```python
from build123d import *

# Parameters (mm, degrees)
F3_D           = 6.2
F3_CSINK_D     = 11
F3_CSINK_ANGLE = 90


with BuildPart() as f1:
    # F0 (on Top) → F1 (revolve)
    with BuildSketch(Plane.XY):
        Polygon((0, 11), (0, 0), (12, 0), (12, 6), (10.5, 6), (9, 4.5), (7.5, 6), (4, 6), (4, 11), align=None)
    revolve(axis=Axis((6, 0, 0), (1, 0, 0)))

    # F3 (through all)
    with Locations(Plane.YZ.offset(12)):
        with Locations((0, 0)):
            CounterSinkHole(F3_D / 2, F3_CSINK_D / 2, counter_sink_angle=F3_CSINK_ANGLE)


solid = f1.part
```
For this review, take the finished solid that the model builds, in its own axes (mm). A direction names the side the tool comes from. Coordinates: 2 decimals unless noted, no trailing zeros. Write each loop counter-clockwise with the first axis right and the second up, starting at its lowest first coordinate (ties: lowest second). Pieces come first, ordered by that corner, then holes. Notation, with made-up numbers: (-27, -30.75) - (-21, -30.75) arc R4 ccw to (-21, -26.75) - close; hole circle Ø5 at (48, 75.25). An arc over 180 degrees is marked (long way). Answer in a Markdown table with one row per item. Add a question column.
Q1. For P1, Ø1.5, axis at y = -4, z = 6.5, coming from the +X side; P2, Ø5.5, axis at y = 0, z = 0, coming from the -X side; P3, Ø1, axis at x = 3, y = 2.5, coming from the -Z side, all flat-tipped, find the tip position at first contact; note any pin that passes through.
Q2. Tool access review of faces 1 (the cylindrical face through (1.97, -2.38, -10.74)), 2 (the cylindrical face through (11, -6, 0)): name each direction out of +Z, -Z, +X, -X, +Y, -Y from which nothing blocks a thin tool from reaching the whole face with its end or side.
Q3. We need section D-D, the plane x = 8. State the section outline as (y, z) points.
Q4. We need section A-A, the plane y = 0. State the section outline as (x, z) points, and give its area (3 significant figures).
Q5. Draft analysis for pull direction Y (two halves, no side actions). For faces 3 (the cylindrical face through (6, -6, 0)), 4 (the conical face through (9.717, 0.697, -3.14)), 5 (the flat face through (12, -3, -5)), state which applies: +Y half, -Y half, draft (parallel to the pull), parting line (faces both ways), or undercut.
Q6. We need section C-C, the plane x = 3.25. State the section outline as (y, z) points, and give its area (3 significant figures).
Q7. For probe 1 along Z at (x, y) = (3, 0); probe 2 along Z at (x, y) = (5.25, 0); probe 3 along X at (y, z) = (-5.75, -6.5), list the stretches that pass through material, from the lowest coordinate up.
Answer list:
| question | item | result |
|---|---|---|
| 1 | P1 | stops at x = 4 |
| 1 | P2 | passes through |
| 1 | P3 | stops at z = -10.82 |
| 2 | face 1 | +X, -X |
| 2 | face 2 | +X |
| 3 | outline | circle Ø11 at (0, 0); hole circle Ø6.2 at (0, 0) |
| 4 | outline | (0, -11) - (4, -11) - (4, -6) - (7.5, -6) - (9, -4.5) - (10.5, -6) - (12, -6) - (12, -5.5) - (9.6, -3.1) - (0, -3.1) - close; (0, 3.1) - (9.6, 3.1) - (12, 5.5) - (12, 6) - (10.5, 6) - (9, 4.5) - (7.5, 6) - (4, 6) - (4, 11) - (0, 11) - close |
| 4 | area | 99.3 mm2 |
| 5 | face 3 | parting line |
| 5 | face 4 | undercut |
| 5 | face 5 | draft |
| 6 | outline | circle Ø22 at (0, 0); hole circle Ø6.2 at (0, 0) |
| 6 | area | 350 mm2 |
| 7 | probe 1 | z = -11 to -3.1, 3.1 to 11 |
| 7 | probe 2 | z = -6 to -3.1, 3.1 to 6 |
| 7 | probe 3 | x = 0 to 4 |
